Solid Edge part; units mm, degrees
sketch "Sketch1" plane through (0, 0, 0) normal (0, 0, 1) x (1, 0, 0)
  circle A0 centre (0, -18.93) radius 3.2
  circle A1 centre (0, 20.92) radius 3.2
  line L0 (9, 30) -> (-9, 30)
  arc A2 (-24, 15) -> (-9, 30) centre (-9, 15) cw
  line L1 (-24, 15) -> (-24, -40)
  line L2 (-24, -40) -> (24, -40)
  line L3 (24, -40) -> (24, 15)
  arc A3 (9, 30) -> (24, 15) centre (9, 15) cw
extrude "Protrusion1" add sketch "Sketch1" against normal blind 5
sketch "Sketch2" plane through (0, -40, -2.5) normal (0, -1, 0) x (1, 0, 0)
  circle A0 centre (-11.5, 17) radius 6.1
  circle A1 centre (11.5, 17) radius 6.1
  arc A2 (24, 17) -> (14.5, 26.5) centre (14.5, 17) ccw
  line L0 (-14.5, 26.5) -> (14.5, 26.5)
  arc A3 (-24, 17) -> (-14.5, 26.5) centre (-14.5, 17) cw
  line L1 (-24, 17) -> (-24, 7.5)
  line L2 (-24, 7.5) -> (-24, -2.5)
  line L3 (-24, -2.5) -> (24, -2.5)
  line L4 (24, -2.5) -> (24, 7.5)
  line L5 (24, 7.5) -> (24, 17)
extrude "Extrusionsausprägung_2" add sketch "Sketch2" along normal blind 5
chamfer "Fase_1" distance 2.54 angle 45 1 edges at (0, -40, 0)
Input: part model. Units: mm. Frame: model coordinates. A direction names the side the tool comes from. Give positions to 0.01 mm unless a question says otherwise; leave off trailing zeros. Order: outer loops, then holes, each group sorted by start corner. A loop starts at its lowest first (then second) coordinate and runs counter-clockwise, first axis right, second up. Notation, with made-up numbers: (-33.75, 78) - (-17.75, 78) arc R20 cw to (-17.75, 108) - close; hole circle Ø2 at (58, -19.75). An arc over 180 degrees is marked (long way). Answer as a JSON object with one key per item and string values. Group by question number.
Q1. Set-up query: faces 5 (the face through (21.143, -42.465, 21.291)), 6 (the face through (0, -3, 0)). Return all of +Z, -Z, +X, -X, +Y, -Y with unobstructed straight access to the full face (end or side cutting, diameter ignored); none if empty.
Q2. Cut plane C-C, the plane z = -3. Output: boundary loops of the cut face in (x, y), then the cut area to 3 significant figures.
Q3. Cut plane B-B, the plane y = -18.93. Output: boundary loops of the cut face in (x, z), then the cut area to 3 significant figures.
Q4. Cut plane A-A, the plane x = 0. Output: boundary loops of the cut face in (y, z), then the cut area to 3 significant figures.
Q5. Cut plane D-D, the plane x = 11.5. Output: boundary loops of the cut face in (y, z), then the cut area to 3 significant figures.
Q6. Mould query, pull axis Z, two halves, no side actions, for faces 1 (the face through (-24, -19.3, -0.3)), 2 (the face through (10.178, -42.465, 20.455)), 3 (the face through (-12.822, -42.465, 20.455)), 4 (the face through (-21.291, -42.465, 21.143)). Classes: pulls with the +Z half, pulls with the -Z half, needs draft (parallel to the pull), parting line crosses it, or undercut.
Q7. Line query: probe 1 along Y at (x, z) = (0, -1.95); probe 2 along Z at (x, y) = (-11.5, -41.25); probe 3 along Y at (x, z) = (6.5, 8). Output: solid intervals per line, ascending.
Q8. First-contact query: pin 1 Ø10.5 at (x, z) = (10, 8.5) entering from +Y; pin 2 Ø3 at (x, y) = (-1.5, -7) entering from +Z; pin 3 Ø8.5 at (x, y) = (0, 20.92) entering from -Z. Flat tips, straight axial feed; report the tip coordinate or a pass-through.
Results:
{
 "1": {"face 5": "+Z, +X, +Y, -Y", "face 6": "+Z, +X, -X, +Y"},
 "2": {"outline": "(-24, -45) - (24, -45) - (24, 15) arc R15 ccw to (9, 30) - (-9, 30) arc R15 ccw to (-24, 15) - close; hole circle Ø6.4 at (0, -18.93); hole circle Ø6.4 at (0, 20.92)", "area": "3,440 mm^2"},
 "3": {"outline": "(-24, -5) - (-3.2, -5) - (-3.2, 0) - (-24, 0) - close; (3.2, -5) - (24, -5) - (24, 0) - (3.2, 0) - close", "area": "208 mm^2"},
 "4": {"outline": "(-45, -5) - (-22.13, -5) - (-22.13, 0) - (-37.46, 0) - (-40, 2.54) - (-40, 24) - (-45, 24) - close; (-15.73, -5) - (17.72, -5) - (17.72, 0) - (-15.73, 0) - close; (24.12, -5) - (30, -5) - (30, 0) - (24.12, 0) - close", "area": "434 mm^2"},
 "5": {"outline": "(-45, -5) - (29.79, -5) - (29.79, 0) - (-37.46, 0) - (-40, 2.54) - (-40, 8.4) - (-45, 8.4) - close; (-45, 20.6) - (-40, 20.6) - (-40, 24) - (-45, 24) - close", "area": "436 mm^2"},
 "6": {"face 1": "needs draft", "face 2": "undercut", "face 3": "undercut", "face 4": "pulls with the +Z half"},
 "7": {"probe 1": "-45 to -22.13, -15.73 to 17.72, 24.12 to 30", "probe 2": "-5 to 8.4, 20.6 to 24", "probe 3": "-45 to -40"},
 "8": {"pin 1": "y = -40", "pin 2": "z = 0", "pin 3": "z = -5"}
}
